For this review, take the finished solid that the model builds, in its own axes (mm). A direction names the side the tool comes from. Give positions to 0.01 mm unless a question says otherwise; leave off trailing zeros. Loops run counter-clockwise (first coordinate to the right, second up) from the corner with the lowest first, then second, coordinate; pieces in that order, holes last. Notation, with made-up numbers: (4.25, 86) -> (14.25, 86) arc R13 cw to (14.25, 93) -> close; hole circle Ø7 at (63, 3.25). An arc over 180 degrees is marked (long way). Write each question's results on one line, items separated by ' | '. Start each with the question number.
```python
from build123d import *

# Parameters (mm, degrees)
EXTRUDE_1_DEPTH     = 3
SKETCH_3_W          = 36
SKETCH_3_H          = 5
EXTRUDE_3_DEPTH     = 6
SKETCH_4_W          = 28
SKETCH_4_H          = 5
EXTRUDE_4_DEPTH     = 14
SKETCH_6_W          = 2
SKETCH_6_H          = 10
EXTRUDE_6_DEPTH     = 10
CHAMFER_1_SIZE      = 10
FILLET_2_R          = 5
SKETCH_12_R         = 2.1
CUT_EXTRUDE_3_DEPTH = 38.802116343
SKETCH_2_R          = 1.1
CUT_EXTRUDE_4_DEPTH = 34.793490497
SKETCH_13_R         = 1.75
CUT_EXTRUDE_5_DEPTH = 2
FILLET_3_R          = 3
FILLET_4_R          = 1


with BuildPart() as part:
    # 草图1 → 凸台-拉伸1 (new body)
    with BuildSketch(Plane(origin=(0, 0, 0), x_dir=(1, 0, 0), z_dir=(0, 1, 0))):
        Polygon((6, 17), (18, 17), (18, -17), (-18, -17), (-18, 17), (-6, 17), (-6, 11), (6, 11), align=None)
    extrude(amount=EXTRUDE_1_DEPTH)

    # 草图3 → 凸台-拉伸3 (add)
    with BuildSketch(Plane(origin=(0, 3, 0), x_dir=(1, 0, 0), z_dir=(0, 1, 0))):
        with Locations((0, -4.5)):
            Rectangle(SKETCH_3_W, SKETCH_3_H)
    extrude(amount=EXTRUDE_3_DEPTH)

    # 草图4 → 凸台-拉伸4 (add)
    with BuildSketch(Plane(origin=(0, 9, 0), x_dir=(1, 0, 0), z_dir=(0, 1, 0))):
        with Locations((0, -4.5)):
            Rectangle(SKETCH_4_W, SKETCH_4_H)
    extrude(amount=EXTRUDE_4_DEPTH)

    # 草图6 → 凸台-拉伸6 (add)
    with BuildSketch(Plane(origin=(0, 3, 0), x_dir=(1, 0, 0), z_dir=(0, 1, 0))):
        with Locations((4, 3)):
            Rectangle(SKETCH_6_W, SKETCH_6_H)
        with Locations((-4, 3)):
            Rectangle(SKETCH_6_W, SKETCH_6_H)
    extrude(amount=EXTRUDE_6_DEPTH)

    # 倒角1
    chamfer_1_edges = [part.edges().sort_by_distance(p)[0] for p in [
        (4, 13, -8),
        (-4, 13, -8),
    ]]
    chamfer(chamfer_1_edges, length=CHAMFER_1_SIZE - 0.0001)  # a hair under: the kernel refuses the full size

    # 圆角2
    fillet_2_edges = [part.edges().sort_by_distance(p)[0] for p in [
        (11.5, 3, 2),
        (0, 3, 2),
        (-11.5, 3, 2),
    ]]
    fillet(fillet_2_edges, radius=FILLET_2_R)

    # 草图12 → 切除-拉伸3 (cut, through all)
    with BuildSketch(Plane.XY.offset(7)):
        with Locations((0, 18)):
            Circle(SKETCH_12_R)
        with Locations((0, 8.5)):
            Circle(SKETCH_12_R)
    extrude(amount=-CUT_EXTRUDE_3_DEPTH, mode=Mode.SUBTRACT)

    # 草图2 → 切除-拉伸4 (cut, through all)
    with BuildSketch(Plane.XZ):
        with Locations(Location((-13.9, 13.9, 0), (0, 0, 270))):
            Circle(SKETCH_2_R)
        with Locations(Location((13.9, 13.9, 0), (0, 0, 270))):
            Circle(SKETCH_2_R)
        with Locations(Location((-13.9, -13.9, 0), (0, 0, 270))):
            Circle(SKETCH_2_R)
        with Locations(Location((13.9, -13.9, 0), (0, 0, 270))):
            Circle(SKETCH_2_R)
    extrude(amount=-CUT_EXTRUDE_4_DEPTH, mode=Mode.SUBTRACT)

    # 草图13 → 切除-拉伸5 (cut)
    with BuildSketch(Plane(origin=(0, 3, 0), x_dir=(1, 0, 0), z_dir=(0, 1, 0))):
        with Locations(Location((-13.9, 13.9, 0), (0, 0, 270))):
            Circle(SKETCH_13_R)
        with Locations(Location((13.9, 13.9, 0), (0, 0, 270))):
            Circle(SKETCH_13_R)
        with Locations(Location((-13.9, -13.9, 0), (0, 0, 270))):
            Circle(SKETCH_13_R)
        with Locations(Location((13.9, -13.9, 0), (0, 0, 270))):
            Circle(SKETCH_13_R)
    extrude(amount=-CUT_EXTRUDE_5_DEPTH, mode=Mode.SUBTRACT)

    # 圆角3
    fillet_3_edges = [part.edges().sort_by_distance(p)[0] for p in [
        (-18, 1.5, -17),
        (18, 1.5, -17),
        (18, 1.5, 17),
        (-18, 1.5, 17),
        (-14, 23, 4.5),
        (14, 23, 4.5),
    ]]
    fillet(fillet_3_edges, radius=FILLET_3_R)

    # 圆角4
    fillet_4_edges = [part.edges().sort_by_distance(p)[0] for p in [
        (18, 9, 4.5),
        (14, 9, 4.5),
        (-18, 9, 4.5),
        (-14, 9, 4.5),
    ]]
    fillet(fillet_4_edges, radius=FILLET_4_R)


solid = part.part
```
1. We need section D-D (z = 13.5). Write out the cut boundary in (x, y), plus the area to 3 significant figures.
2. We need section B-B (x = 0). Write out the cut boundary in (y, z).
3. Wall thickness on L1, parallel to X at y = 2.15, z = 13.9; L2, parallel to X at y = 2.5, z = -13.5; L3, parallel to Z at x = -1, y = 12.5: over which ranges is each line inside the solid? List them lowest first.
4. We need section A-A (y = 18). Write out the cut boundary in (x, z), plus the area to 3 significant figures.
5. Draft analysis for pull direction X (two halves, no side actions). For faces 1 (the flat face through (-11, 1, -17)), 2 (the cylindrical face through (-14.301, 9.285, 4.465)), 3 (the flat face through (5, 7, -2)), 4 (the cylindrical face through (0, 4, 0)), state which applies: released by +X, released by -X, zero draft, split by the parting line, or undercut.
6. For pin 1 Ø4 at (x, z) = (-13, 13.5) entering from +Y; pin 2 Ø6 at (x, y) = (6, 16.5) entering from +Z; pin 3 Ø1 at (x, y) = (-5, 20.5) entering from -Z, all flat-tipped, find the tip position at first contact; note any pin that passes through.
7. Machinability: for faces 5 (the flat face through (0, 3, 12)), 6 (the flat face through (-6, 1, -14)), 7 (the flat face through (-14, 15, 5)), 8 (the flat face through (0, 15, 2)), which of the approach directions +Z, -Z, +X, -X, +Y, -Y give a long, thin tool a straight path to every point of the face, cutting with its end or side? Answer none if there is none.
Response:
1) outline: (-18, 0) -> (-14.92, 0) -> (-14.92, 1) -> (-15.6, 1) -> (-15.6, 3) -> (-18, 3) -> close; (-12.88, 0) -> (12.88, 0) -> (12.88, 1) -> (12.2, 1) -> (12.2, 3) -> (-12.2, 3) -> (-12.2, 1) -> (-12.88, 1) -> close; (14.92, 0) -> (18, 0) -> (18, 3) -> (15.6, 3) -> (15.6, 1) -> (14.92, 1) -> close | area: 90.3 mm2
2) outline: (0, -11) -> (3, -11) -> (3, -3) arc R5 cw to (6.4, 1.74) -> (6.4, 7) -> (3, 7) -> (3, 17) -> (0, 17) -> close; (10.6, 2) -> (15.9, 2) -> (15.9, 7) -> (10.6, 7) -> close; (20.1, 2) -> (23, 2) -> (23, 7) -> (20.1, 7) -> close
3) L1: x = -18 to -15.65, -12.15 to 12.15, 15.65 to 18 | L2: x = -18 to -15.6, -12.2 to -6, 6 to 12.2, 15.6 to 18 | L3: z = 2 to 7
4) outline: (-14, 2) -> (-2.1, 2) -> (-2.1, 7) -> (-14, 7) -> close; (2.1, 2) -> (14, 2) -> (14, 7) -> (2.1, 7) -> close | area: 119 mm2
5) face 1: zero draft | face 2: released by -X | face 3: released by +X | face 4: undercut
6) pin 1: stops at y = 3 | pin 2: stops at z = 7 | pin 3: stops at z = 2
7) face 5: +Z, +X, -X, +Y | face 6: -Z, +Y, -Y | face 7: +Z, -Z, -X, +Y | face 8: -Z, +Y
